Here's the drawing with two shaded views (mm, measured from the low corner). I have some questions. A direction names the side the tool comes from. Coordinates: 2 decimals unless noted, no trailing zeros. Write each loop counter-clockwise with the first axis right and the second up, starting at its lowest first coordinate (ties: lowest second). Pieces come first, ordered by that corner, then holes.
Item 1: I want a section at B-B on z = 2.25. Please give me the cut outline in (x, y), then the cut area to 3 significant figures.
Item 2: I want a section at A-A on y = 12.5. Please give me the cut outline in (x, z).
Item 3: I want a section at C-C on x = 3. Please give me the cut outline in (y, z).
Item 4: If I drill on probe 1 along Y at (x, z) = (6, 9.75), over which ranges is the centre line in solid material (lowest first)?
Item 5: Which directions (+Z, -Z, +X, -X, +Y, -Y) give clear straight access to the entire face, cutting with the end or side of a thin tool? Please do the marked faces 1 and 2.
Item 6: For P1, Ø4, axis at y = 10, z = 6, coming from the +X side; P2, Ø6, axis at x = 3, y = 6.5, coming from the -Z side; P3, Ø1.5, axis at x = 9, z = 5, coming from the +Y side, each with a flat end and sliding along its axis, tell me the tip position at first contact or that it passes through.
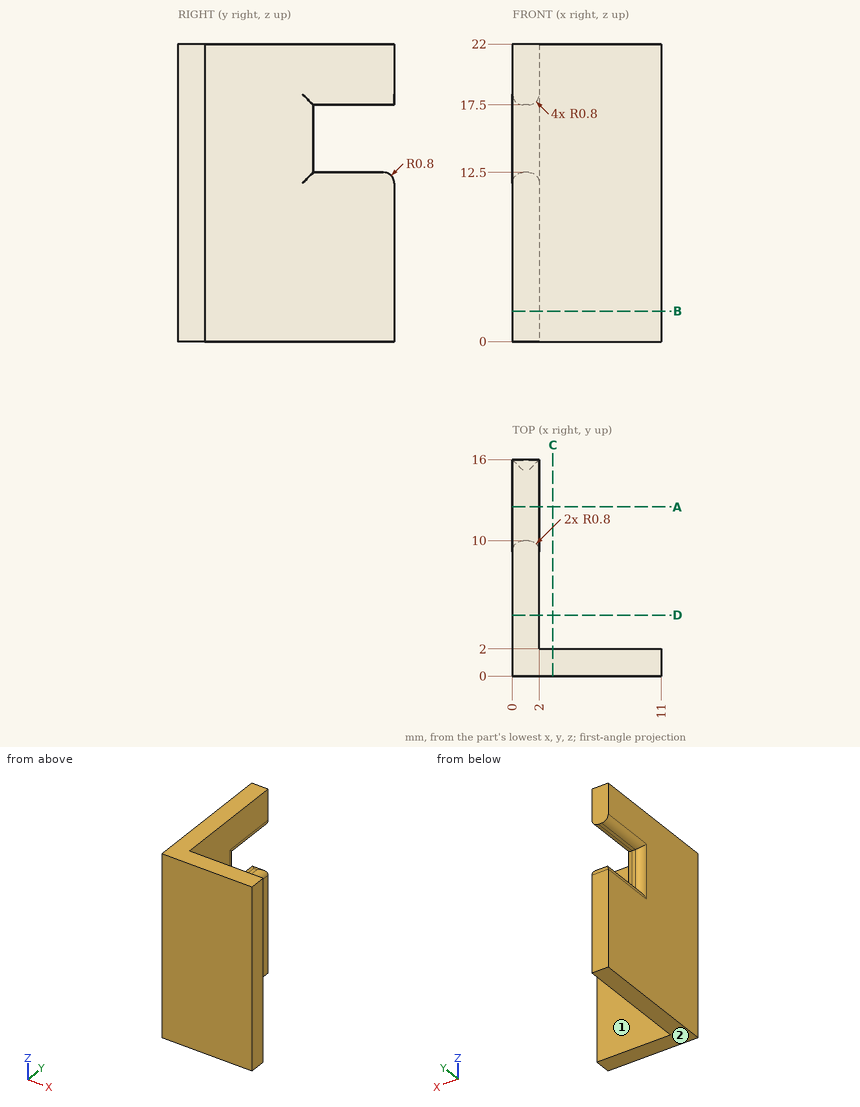
Response values:
1. outline: (0, 0) - (11, 0) - (11, 2) - (2, 2) - (2, 16) - (0, 16) - close
1. area: 50.0 mm2
2. outline: (0, 0) - (2, 0) - (2, 11.7) arc R0.8 ccw to (1.2, 12.5) - (0.8, 12.5) arc R0.8 ccw to (0, 11.7) - close; (0, 18.3) arc R0.8 ccw to (0.8, 17.5) - (1.2, 17.5) arc R0.8 ccw to (2, 18.3) - (2, 22) - (0, 22) - close
3. outline: (0, 0) - (2, 0) - (2, 22) - (0, 22) - close
4. probe 1: y = 0 to 2
5. face 1: +Z, -Z, +X, +Y
5. face 2: -Z, +X, -X, +Y, -Y
6. P1: stops at x = 2
6. P2: stops at z = 0
6. P3: stops at y = 2
